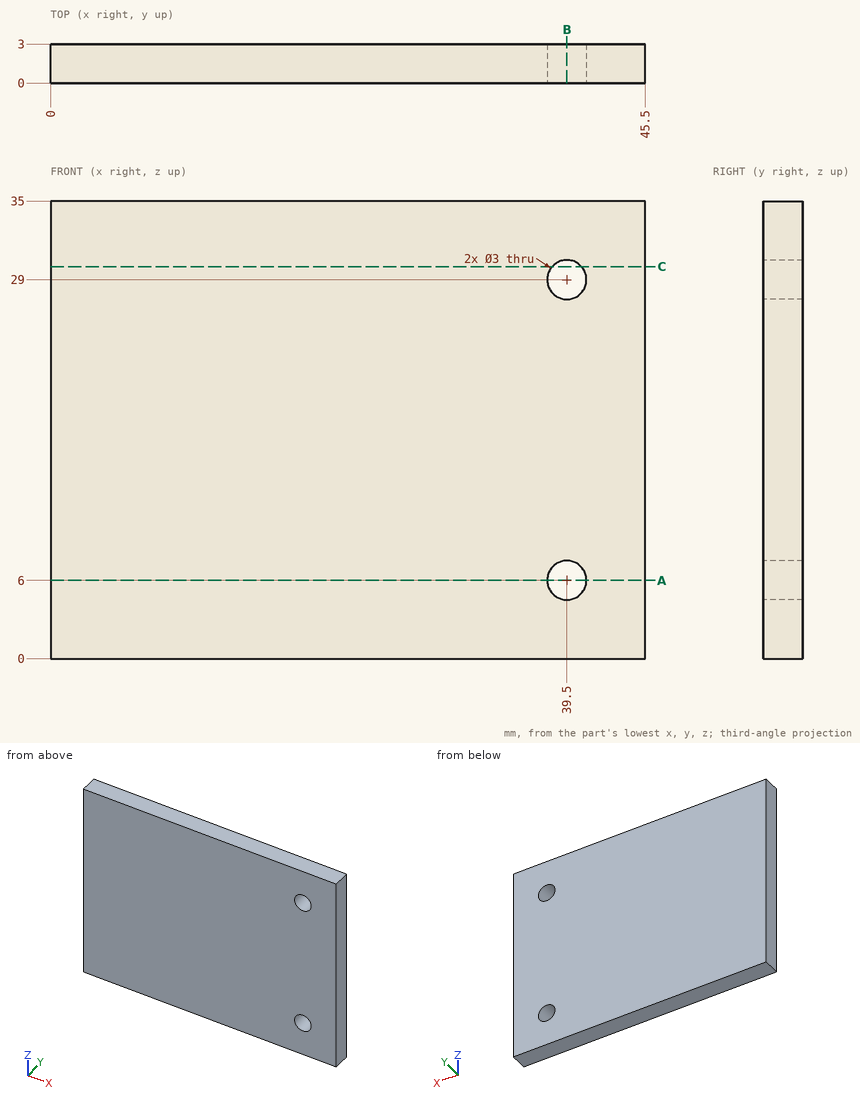
Here's the drawing with two shaded views (mm, measured from the low corner). I have some questions. Coordinates: 2 decimals unless noted, no trailing zeros. Write each loop counter-clockwise with the first axis right and the second up, starting at its lowest first coordinate (ties: lowest second). Pieces come first, ordered by that corner, then holes. Notation, with made-up numbers: (22, -4.5) -> (69, -4.5) arc R21 ccw to (69, 27.5) -> close; hole circle Ø4 at (88.5, -6). An arc over 180 degrees is marked (long way). Answer as CSV lines item,"result".
1) If we section it at A-A on z = 6: Please give me the cut outline in (x, y), then the cut area to 4 significant figures.
Check result:
outline,"(0, 0) -> (38, 0) -> (38, 3) -> (0, 3) -> close; (41, 0) -> (45.5, 0) -> (45.5, 3) -> (41, 3) -> close"
area,"127.5 mm²"
2) Will this pin go through, and if not, where does the flat tip stop? P1, Ø2.5, axis at x = 39.5, z = 6, coming from the +Y side.
Check result:
P1,"through"
3) If we section it at C-C on z = 30: Please give me the cut outline in (x, y), then the cut area to 3 significant figures.
Check result:
outline,"(0, 0) -> (38.38, 0) -> (38.38, 3) -> (0, 3) -> close; (40.62, 0) -> (45.5, 0) -> (45.5, 3) -> (40.62, 3) -> close"
area,"130 mm²"
4) If I drill on line 1 (Z direction, x = 39.5, y = 1.8); line 2 (X direction, y = 2.25, z = 29), over which ranges is the centre line in solid material (lowest first)? Write a range as from..to.
Check result:
line 1,"0..4.5, 7.5..27.5, 30.5..35"
line 2,"0..38, 41..45.5"
5) If we section it at B-B on x = 39.5: Please give me the cut outline in (y, z), then the cut area to 3 significant figures.
Check result:
outline,"(0, 0) -> (3, 0) -> (3, 4.5) -> (0, 4.5) -> close; (0, 7.5) -> (3, 7.5) -> (3, 27.5) -> (0, 27.5) -> close; (0, 30.5) -> (3, 30.5) -> (3, 35) -> (0, 35) -> close"
area,"87.0 mm²"
